```python
from build123d import *

# Parameters (mm, degrees)
ABRAZADERA_PROFILE_R         = 19
BRAZO_PROFILE_R              = 5
PLACA_INT_PROFILE_R          = 3
PLACA_EXT_PROFILE_R          = 3
PUENTE_PLACAS_PROFILE_R      = 3
TALADRO_ABRAZADERA_PROFILE_R = 15.9


with BuildPart() as part:
    # Abrazadera: sweep along a curve in space
    with BuildLine() as abrazadera_path:
        Line((-51.165048326, 167.353332294, 0), (-57.012482421, 186.479427413, 0))
    # Abrazadera profile (on start of the path) → Abrazadera (sweep)
    with BuildSketch(Plane(origin=(-51.165048326, 167.353332294, 0), x_dir=(0.9563047559630354, 0.29237170472273677, 0), z_dir=(-0.29237170472273677, 0.9563047559630354, 0))):
        Circle(ABRAZADERA_PROFILE_R)
    sweep(path=abrazadera_path.line)

    # Brazo: sweep along a curve in space
    with BuildLine() as brazo_path:
        Line((-54.088765374, 176.916379853, 15), (-20, 120, 50))
    # Brazo profile (on start of the path) → Brazo (sweep)
    with BuildSketch(Plane(origin=(-54.088765374, 176.916379853, 15), x_dir=(0, -0.523820970586938, -0.851828381056512), z_dir=(0.45445554568660007, -0.7587826716841304, 0.4666037013854347))):
        Circle(BRAZO_PROFILE_R)
    sweep(path=brazo_path.line)

    # Placa_ext: sweep along a curve in space
    with BuildLine() as placa_ext_path:
        Line((-50, 118, 50), (10, 122, 50))
    # Placa_ext profile (on start of the path) → Placa_ext (sweep)
    with BuildSketch(Plane(origin=(-50, 118, 50), x_dir=(-0.06651901052377393, 0.9977851578566089, 0), z_dir=(0.9977851578566089, 0.06651901052377393, 0))):
        Circle(PLACA_EXT_PROFILE_R)
    sweep(path=placa_ext_path.line)



with BuildPart() as body_2:
    # Placa_int: sweep along a curve in space
    with BuildLine() as placa_int_path:
        Line((-50, 118, 37), (10, 122, 37))
    # Placa_int profile (on start of the path) → Placa_int (sweep)
    with BuildSketch(Plane(origin=(-50, 118, 37), x_dir=(-0.06651901052377393, 0.9977851578566089, 0), z_dir=(0.9977851578566089, 0.06651901052377393, 0))):
        Circle(PLACA_INT_PROFILE_R)
    sweep(path=placa_int_path.line)


with BuildPart() as part_1:
    add(part.part)

    add(body_2.part)  # Puente_placas merges body 2
    # Puente_placas: sweep along a curve in space
    with BuildLine() as puente_placas_path:
        Line((-50, 118, 37), (-50, 118, 50))
    # Puente_placas profile (on start of the path) → Puente_placas (sweep)
    with BuildSketch(Plane(origin=(-50, 118, 37), x_dir=(1, 0, 0), z_dir=(0, 0, 1))):
        Circle(PUENTE_PLACAS_PROFILE_R)
    sweep(path=puente_placas_path.line)

    # Taladro_abrazadera: sweep along a curve in space
    with BuildLine() as taladro_abrazadera_path:
        Line((-49.703189803, 162.571808514, 0), (-58.474340945, 191.260951193, 0))
    # Taladro_abrazadera profile (on start of the path) → Taladro_abrazadera (sweep, cut)
    with BuildSketch(Plane(origin=(-49.703189803, 162.571808514, 0), x_dir=(0.9563047559630354, 0.2923717047227367, 0), z_dir=(-0.2923717047227367, 0.9563047559630354, 0))):
        Circle(TALADRO_ABRAZADERA_PROFILE_R)
    sweep(path=taladro_abrazadera_path.line, mode=Mode.SUBTRACT)


solid = part_1.part
```
Work out the finished part from the listing and answer in its coordinate system (mm). A direction names the side the tool comes from. Give positions to 0.01 mm unless a question says otherwise; leave off trailing zeros. Loops run counter-clockwise (first coordinate to the right, second up) from the corner with the lowest first, then second, coordinate; pieces in that order, holes last. Notation, with made-up numbers: M 71,-24 L 80,-24 A24 ccw 80,5 Z; hole C 58.5,-5.5 d8. An arc over 180 degrees is marked long. One line per item, written item: value. Start each with the question number.
1. Find section A-A (z = 12). Give the vertices of the cut face in (x, y), and give its area (3 significant figures).
2. Determine the mould class of faces 5 (the face through (-49.022, 188.922, 13.985)), 6 (the face through (-19.4, 117.8, 52)), 7 (the face through (-51, 118, 50)) for opening direction Z: released by +Z, released by -Z, zero draft, split by the parting line, or undercut.
3. Each of these flat-tipped pins is pushed along its axis until it touches: P1, Ø2, axis at y = 167.5, z = 5, coming from the -X side; P2, Ø5, axis at y = 147, z = 40.5, coming from the +X side; P3, Ø2.5, axis at x = -51, y = 116.5, coming from the -Z side. Where does it stop, or does it pass through?
4. Find the intervals of material crossed by probe 1 along X at (y, z) = (173, 9.5); probe 2 along Z at (x, y) = (-67.5, 174); probe 3 along Z at (x, y) = (-31.5, 143), in increasing order.
5. Which of the six approach directions +Z, -Z, +X, -X, +Y, -Y give full straight-line access (tool end or side, diameter ignored) to faces 1 (the face through (-53, 118, 44)), 2 (the face through (-50, 118, 51)), 3 (the face through (-50, 118, 36)), 4 (the face through (10, 122, 37))?
Reported:
1. outline: M -71.1,182.17 L -65.25,163.05 L -61.14,164.3 L -66.99,183.43 Z; M -47.04,189.53 L -41.19,170.4 L -37.08,171.66 L -42.93,190.79 Z
1. area: 172 mm²
2. face 5: zero draft
2. face 6: undercut
2. face 7: released by +Z
3. P1: stops at x = -70.78
3. P2: stops at x = -30.06
3. P3: stops at z = 34.12
4. probe 1: x = -70.1 to -66.22, -39.56 to -35.69
4. probe 2: z = -13.19 to -8.11, 8.11 to 13.19
4. probe 3: z = 31.27 to 41.68
5. face 1: none
5. face 2: +Z, -X, -Y
5. face 3: -Z, -X, -Y
5. face 4: +Z, -Z, +X, +Y
